Autodesk Inventor part; units mm, degrees
ref_plane "YZ Plane" through (0, 0, 0) normal (1, 0, 0) x (0, 1, 0)
ref_plane "XZ Plane" through (0, 0, 0) normal (0, 1, 0) x (-1, 0, 0)
ref_plane "XY Plane" through (0, 0, 0) normal (0, 0, 1) x (1, 0, 0)
sketch "Sketch1" plane through (0, 0, 0) normal (0, 0, 1) x (1, 0, 0)
  line L0 (0, 0) -> (80, 0)
  line L1 (80, 0) -> (80, 125.359)
  line L2 (60, 200) -> (80, 125.359)
  line L3 (60, 200) -> (137.2741, 200) construction
  line L4 (0, 0) -> (0, 125.359)
  line L5 (20, 200) -> (0, 125.359)
  line L6 (84, 125.8856) -> (84, -4)
  line L7 (84, -4) -> (-4, -4)
  line L8 (-4, -4) -> (-4, 125.8856)
  line L9 (-4, 125.8856) -> (16.9307, 204)
  line L10 (63.0693, 204) -> (84, 125.8856)
  line L11 (20, 204) -> (20, 200)
  line L12 (60, 200) -> (60, 204)
  line L13 (16.9307, 204) -> (20, 204)
  line L14 (60, 204) -> (63.0693, 204)
  point P0 (40, 0)
  dimension "d0" = 80
  dimension "d4" = 75
  dimension "d5" = 4
extrude "Extrusion1" add sketch "Sketch1" along normal blind 70
sketch "Sketch2" plane through (0, 0, 0) normal (0, 0, -1) x (-1, 0, 0)
  line L0 (-16.9307, 204) -> (4, 125.8856)
  line L1 (-84, 125.8856) -> (-63.0693, 204)
  line L2 (-16.9307, 204) -> (-63.0693, 204)
  line L3 (-80, 125.359) -> (-80, 0)
  line L4 (-60, 200) -> (-80, 125.359)
  line L5 (-60, 204) -> (-60, 200)
  line L6 (-63.0693, 204) -> (-60, 204)
  line L7 (-84, 125.8856) -> (-63.0693, 204)
  line L8 (-84, -4) -> (-84, 125.8856)
  line L9 (4, -4) -> (-84, -4)
  line L10 (4, 125.8856) -> (4, -4)
  line L11 (-16.9307, 204) -> (4, 125.8856)
  line L12 (-20, 204) -> (-16.9307, 204)
  line L13 (-20, 200) -> (-20, 204)
  line L14 (0, 125.359) -> (-20, 200)
  line L15 (0, 0) -> (0, 125.359)
  line L16 (-80, 0) -> (0, 0)
extrude "Extrusion2" add sketch "Sketch2" along normal blind 3
chamfer "Chamfer1" distance 5 angle 45 5 edges at (40, -4, -3) (84, 60.9428, -3) (-4, 60.9428, -3) (6.4653, 164.9428, -3) (73.5347, 164.9428, -3)
chamfer "Chamfer2" distance 3 angle 45 7 edges at (20, 202, 0) (10, 162.6795, 0) (60, 202, 0) (70, 162.6795, 0) (80, 62.6795, 0) (0, 62.6795, 0) (40, 0, 0)
chamfer "Chamfer3" distance 3 angle 45 4 edges at (84, -4, 36) (-4, -4, 36) (0, 0, 36.5) (80, 0, 36.5)
sketch "Sketch3" plane through (0, 0, 70) normal (0, 0, 1) x (1, 0, 0)
  line L0 (77, 0) -> (78.5, 1.5)
  line L1 (81, -4) -> (82.5, -2.5)
  line L2 (78.5, 1.5) -> (82.5, -2.5)
  line L3 (79, 1) -> (82.5, -2.5)
  circle A0 centre (80.75, -0.75) radius 1
  line L4 (-4, -1) -> (-2.5, -2.5)
  line L5 (-2.5, -2.5) -> (1.5, 1.5)
  line L6 (0, 3) -> (3, 0)
  line L7 (1, 1) -> (-2.5, -2.5)
  circle A1 centre (-0.75, -0.75) radius 1
  line L8 (3, 124.964) -> (0, 125.359)
  line L9 (16.9307, 204) -> (-4, 125.8856)
  line L10 (80, 125.359) -> (77, 124.964)
  line L11 (84, -1) -> (84, 125.8856)
  line L12 (1, 125.2273) -> (-4, 125.8856)
  circle A2 centre (82, 125.6223) radius 1
  circle A3 centre (-2, 125.6223) radius 1
  point P0 (0, 0)
  dimension "d19" = 2
  dimension "d20" = 2
  dimension "d22" = 2
  dimension "d23" = 2
extrude "Extrusion3" cut sketch "Sketch3" against normal blind 5
sketch "Sketch4" plane through (22.1071, 204, -3) normal (0, 1, 0) x (1, 0, 0)
  line L0 (35.7859, 0) -> (40.9622, -5)
  line L1 (38.374, -2.5) -> (36.3929, -4.5)
  line L2 (34.8929, -3) -> (37.8929, -6)
  circle A0 centre (37.3835, -3.5) radius 1
  line L3 (-21.1071, 0) -> (56.8929, 0)
  line L4 (17.8929, 0) -> (17.8929, -26)
  circle A1 centre (-1.5976, -3.5) radius 1
  point P0 (-22.1071, -3)
  dimension "d26" = 2
extrude "Extrusion4" cut sketch "Sketch4" against normal blind 15
sketch "Sketch5" plane through (0, 0, 0) normal (0, 0, 1) x (1, 0, 0)
  line L0 (77, 3) -> (3, 3)
  line L1 (40, 3) -> (40, 43)
  line L2 (40, 43) -> (40, 113)
  line L3 (40, 78) -> (20, 78)
  line L4 (20, 78) -> (20, 55.5)
  line L5 (20, 55.5) -> (60, 55.5)
  line L6 (60, 55.5) -> (60, 100.5)
  line L7 (60, 100.5) -> (20, 100.5)
  line L8 (20, 100.5) -> (20, 78)
  line L9 (40, 78) -> (70, 78)
  line L10 (70, 78) -> (70, 98)
  circle A0 centre (70, 98) radius 1
  line L11 (70, 78) -> (70, 58)
  circle A1 centre (70, 58) radius 1
  circle A2 centre (10, 98) radius 1
  circle A3 centre (10, 58) radius 1
  line L12 (40, 113) -> (40, 133)
  line L13 (40, 133) -> (63.1521, 133)
  line L14 (63.1521, 133) -> (63.1521, 155.7076)
  circle A4 centre (63.1521, 155.7076) radius 1.5
  circle A5 centre (63.1521, 133) radius 1.5
  circle A6 centre (16.8479, 155.7076) radius 1.5
  circle A7 centre (16.8479, 133) radius 1.5
  point P0 (0, 0)
  dimension "d29" = 40
  dimension "d30" = 70
  dimension "d31" = 20
  dimension "d32" = 22.5
  dimension "d33" = 40
  dimension "d34" = 45
  dimension "d35" = 30
  dimension "d36" = 20
  dimension "d37" = 2
  dimension "d38" = 20
  dimension "d39" = 2
  dimension "d40" = 20
  dimension "d41" = 23.1521
  dimension "d42" = 22.7076
  dimension "d43" = 3
  dimension "d44" = 3
extrude "Extrusion5" cut sketch "Sketch5" against normal blind 40
sketch "Sketch7" plane through (-1, -4, 2) normal (0, -1, 0) x (1, 0, 0)
  line L0 (78, 68) -> (4, 68)
  line L1 (41, 68) -> (41, 34)
  line L2 (54.7, 34) -> (27.3, 34)
  line L3 (54.7, 34) -> (54.7, 20.8)
  line L4 (54.7, 20.8) -> (27.3, 20.8)
  line L5 (27.3, 34) -> (27.3, 20.8)
  point P0 (1, -2)
  dimension "d47" = 27.4
  dimension "d48" = 34
  dimension "d49" = 13.2
extrude "Extrusion6" cut sketch "Sketch7" against normal blind 27.4
sketch "Sketch8" plane through (-4, 125.8856, 2) normal (-0.9659258, 0.258819, 0) x (0, 0, 1)
  line L0 (-2, 13.7678) -> (-2, 10.7678)
  line L1 (-2, 35.7017) -> (-2, 32.7017)
  line L2 (3.9828, 34.5121) -> (3.9828, 12.5782)
  line L3 (3.9828, 23.5451) -> (5.9828, 23.5451)
  line L4 (5.9828, 23.5451) -> (12.9828, 23.5451)
  line L5 (12.9828, 23.5451) -> (12.9828, 30.2951)
  line L6 (12.9828, 30.2951) -> (12.9828, 16.7951)
  line L7 (12.9828, 16.7951) -> (5.9828, 16.7951)
  line L8 (5.9828, 16.7951) -> (5.9828, 29.9848)
  line L9 (5.9828, 29.9848) -> (12.9828, 30.2951)
  point P0 (-2, -120.5609)
  point P1 (12.9828, 30.2951)
  dimension "d52" = 2
  dimension "d53" = 7
  dimension "d54" = 6.75
  dimension "d55" = 13.5
extrude "Extrusion7" cut sketch "Sketch8" against normal blind 9
chamfer "Chamfer4" distance 1 angle 45 4 edges at (5.7728, 154.6308, 14.9828) (2.2788, 141.5908, 14.9828) (2.2788, 141.5908, 7.9828) (5.6925, 154.331, 7.9828)
sketch "Sketch9" plane through (-4, 125.8856, 2) normal (-1, 0, 0) x (0, 0, 1)
  line L0 (1, -0.5266) -> (1, -122.8856)
  line L1 (1, -48.8247) -> (7.6436, -48.8247)
  line L2 (7.6436, -48.8247) -> (7.6436, -34.3247)
  line L3 (7.6436, -34.3247) -> (7.6436, -63.3247)
  circle A0 centre (7.6436, -34.3247) radius 2
  circle A1 centre (7.6436, -63.3247) radius 2
  point P0 (-2, -125.8856)
  dimension "d61" = 14.5
  dimension "d62" = 29
  dimension "d63" = 4
  dimension "d64" = 4
extrude "Extrusion8" cut sketch "Sketch9" against normal blind 999
sketch "Sketch17" plane through (0, 0, -3) normal (0, 0, -1) x (-1, 0, 0)
  line L0 (-60, 55.5) -> (-60, 100.5)
  line L1 (-60, 78) -> (-77, 78)
  line L2 (-77, 124.964) -> (-77, 3)
  line L3 (-77, 78) -> (-77, 43)
  line L4 (-77, 78) -> (-77, 113)
  line L5 (-60, 55.5) -> (-20, 55.5)
  line L6 (-40, 55.5) -> (-40, 37.7198)
  line L7 (-20, 55.5) -> (-20, 100.5)
  line L8 (-20, 78) -> (-3, 78)
  line L9 (-3, 78) -> (-3, 43)
  line L10 (-3, 78) -> (-3, 113)
  line L11 (-20, 55.5) -> (-60, 55.5)
  line L12 (-77, 43) -> (-3, 43)
  line L13 (-3, 3) -> (-3, 124.964)
  line L14 (-3, 113) -> (-77, 113)
  line L15 (-79, 1) -> (-79, 125.2273)
  circle A0 centre (-63.1521, 133) radius 1.5
  circle A1 centre (-70, 98) radius 1
  circle A2 centre (-10, 58) radius 1
  circle A3 centre (-16.8479, 133) radius 1.5
  circle A4 centre (-63.1521, 155.7076) radius 1.5
  circle A5 centre (-70, 58) radius 1
  circle A6 centre (-10, 98) radius 1
  circle A7 centre (-16.8479, 155.7076) radius 1.5
  line L16 (-20, 55.5) -> (-60, 55.5)
  line L17 (-60, 55.5) -> (-60, 100.5)
  line L18 (-60, 100.5) -> (-20, 100.5)
  line L19 (-20, 100.5) -> (-20, 55.5)
  line L20 (-79, 125.2273) -> (-57.8929, 204)
  line L21 (-79, 1) -> (-79, 125.2273)
  line L22 (-1, 1) -> (-79, 1)
  line L23 (-1, 125.2273) -> (-1, 1)
  line L24 (-22.1071, 204) -> (-1, 125.2273)
  line L25 (-22.1071, 204) -> (-57.8929, 204)
  point P0 (0, 0)
  dimension "d106" = 35
  dimension "d107" = 35
extrude "Extrusion16" add sketch "Sketch17" along normal blind 3 contours L5 L6 L12 L2 L1 L0 | L0 L18 L7 L5 | L1 L2 L14 L10 L8 L7 L18 L0 | L5 L7 L8 L9 L12 L6
sketch "Sketch18" plane through (0, 0, 70) normal (0, 0, 1) x (1, 0, 0)
  line L0 (-145.0841, -156.9657) -> (0, 339.906)
  line L1 (0, 339.906) -> (209.9789, 212.1699)
  line L2 (209.9789, 212.1699) -> (104.9894, -207.8436)
  line L3 (104.9894, -207.8436) -> (-145.0841, -156.9657)
  point P0 (0, 0)
extrude "Extrusion17" cut sketch "Sketch18" against normal blind 73
sketch "Sketch19" plane through (0, 0, -3) normal (0, 0, 1) x (1, 0, 0)
  line L0 (3, 113) -> (77, 113)
  line L1 (77, 43) -> (3, 43)
  line L2 (40, 43) -> (40, 113)
  line L3 (40, 78) -> (25, 78)
  line L4 (25, 78) -> (25, 63)
  line L5 (25, 63) -> (40, 63)
  line L6 (40, 63) -> (55, 63)
  line L7 (55, 63) -> (55, 93)
  line L8 (55, 93) -> (25, 93)
  line L9 (25, 93) -> (25, 78)
  line L10 (22, 78) -> (22, 60)
  line L11 (22, 60) -> (40, 60)
  line L12 (40, 60) -> (58, 60)
  line L13 (58, 60) -> (58, 96)
  line L14 (58, 96) -> (22, 96)
  line L15 (22, 96) -> (22, 78)
  point P0 (0, 0)
  dimension "d112" = 15
  dimension "d113" = 15
  dimension "d114" = 15
  dimension "d115" = 15
  dimension "d116" = 30
  dimension "d117" = 3
extrude "Extrusion18" add sketch "Sketch19" along normal blind 73 contours L11 L10 L15 L14 L2 L8 L9 L4 L5 | L2 L6 L7 L8 L14 L13 L12
sketch "Sketch20" plane through (0, 0, -3) normal (0, 0, 1) x (1, 0, 0)
  line L0 (25, 93) -> (25, 63)
  line L1 (25, 63) -> (55, 63)
  line L2 (55, 63) -> (55, 93)
  line L3 (55, 93) -> (25, 93)
  point P0 (0, 0)
extrude "Extrusion19" cut sketch "Sketch20" against normal blind 73
chamfer "Chamfer7" distance 3 angle 45 8 edges at (58, 60, 33.5) (25, 93, 32) (58, 96, 33.5) (55, 63, 32) (22, 96, 33.5) (55, 93, 32) (25, 63, 32) (22, 60, 33.5)
chamfer "Chamfer8" distance 3 angle 45 4 edges at (3, 78, -3) (40, 43, -3) (77, 78, -3) (40, 113, -3)
sketch "Sketch21" plane through (25, 96, -3) normal (0, 1, 0) x (1, 0, 0)
  line L0 (0, -73) -> (0, 0)
  line L1 (30, -73) -> (0, -73)
  line L2 (30, 0) -> (30, -73)
  line L3 (0, 0) -> (30, 0)
  line L4 (0, -73) -> (0, 3)
  line L5 (0, -35) -> (30, -35)
  line L6 (30, -73) -> (30, 0)
  circle A0 centre (15, -35) radius 9.425
  point P0 (-25, -3)
  dimension "d128" = 18.85
extrude "Extrusion20" cut sketch "Sketch21" against normal blind 3 contours A0 L5 | L5 A0
sketch "Sketch22" plane through (0, 0, 70) normal (0, 0, 1) x (1, 0, 0)
  line L0 (25, 60) -> (22, 63)
  line L1 (25, 60) -> (55, 60)
  line L2 (58, 63) -> (55, 60)
  line L3 (58, 63) -> (58, 93)
  line L4 (55, 96) -> (58, 93)
  line L5 (55, 96) -> (25, 96)
  line L6 (22, 93) -> (25, 96)
  line L7 (22, 93) -> (22, 63)
  line L8 (28, 93) -> (52, 93)
  line L9 (55, 90) -> (52, 93)
  line L10 (55, 90) -> (55, 66)
  line L11 (52, 63) -> (55, 66)
  line L12 (52, 63) -> (28, 63)
  line L13 (25, 66) -> (28, 63)
  line L14 (25, 66) -> (25, 90)
  line L15 (28, 93) -> (25, 90)
  line L16 (25, 90) -> (28, 93)
  line L17 (26.5, 91.5) -> (23.5, 94.5)
  line L18 (22, 93) -> (25, 96)
  line L19 (25, 60) -> (22, 63)
  line L20 (23.5, 61.5) -> (26.5, 64.5)
  line L21 (28, 63) -> (25, 66)
  line L22 (56.5, 61.5) -> (53.5, 64.5)
  line L23 (53.5, 91.5) -> (56.5, 94.5)
  line L24 (58, 93) -> (55, 96)
  circle A0 centre (25, 63) radius 1
  circle A1 centre (55, 63) radius 1
  circle A2 centre (55, 93) radius 1
  circle A3 centre (25, 93) radius 1
  point P0 (0, 0)
  dimension "d131" = 2
  dimension "d132" = 2
  dimension "d133" = 2
  dimension "d134" = 2
extrude "Extrusion21" cut sketch "Sketch22" against normal blind 20 contours A0 L20 | L20 A0 | A1 L22 | L22 A1 | A3 L17 | L17 A3 | A2 L23 | L23 A2
equation "\"d45\" = d33"
equation "\"d50\" = d47"
properties part number "the handle"
Model file for the job. Use its own axes, mm. A direction names the side the tool comes from. Coordinates: 2 decimals unless noted, no trailing zeros. Loops run counter-clockwise (first coordinate to the right, second up) from the corner with the lowest first, then second, coordinate; pieces in that order, holes last. Notation, with made-up numbers: (63.25, 75) - (117.25, 75) arc R15 cw to (117.25, 86) - close; hole circle Ø7 at (73, 26). An arc over 180 degrees is marked (long way). Answer as a JSON object with one key per item and string values. Group by question number.
(1) Cut at C-C (z = 55). Give the cut face in (x, y), then the cut area to 3 significant figures.
(2) Flat gauge pins, fed straight in: pin 1 (1.2 mm diameter, centred on x = 55, y = 63, fed in from +Z); pin 2 (15 mm diameter, centred on x = 42.5, z = 30.5, fed in from -Y); pin 3 (7 mm diameter, centred on y = 74, z = 14.5, fed in from +X); pin 4 (1.6 mm diameter, centred on x = 10, y = 98, fed in from -Z). Where does each tip first touch, or does it go through?
(3) Cut at B-B (x = 40). State how many separate pieces and enclosed holes the cut face has, then the cut area to 3 significant figures.
(4) Tool access for faces 4 (the face through (55, 78, 33)), 5 (the face through (56, 95, 34)), 6 (the face through (5, 78, -4)), 7 (the face through (25, 93, 50)), 8 (the face through (39, 111, -4)): list every direction of +Z, -Z, +X, -X, +Y, -Y with a clear straight run to the whole face (end or side of a thin tool).
(5) Two-plate mould, pull along X, no slides. Class faces 1 (the face through (54, 91, 31)), 2 (the face through (22, 78, 33)), 3 (the face through (41, 94, -6)): released by +X, released by -X, zero draft, split by the parting line, or undercut.
(6) Probe line 1 along Y through (x, z) = (32, 57); line 2 along X through (y, z) = (73, 15.5); line 3 along Y through (x, z) = (70, -5). List the from-to ranges inside material, lowest first.
Geometry says:
{
 "1": {"outline": "(22, 63) - (25, 60) - (55, 60) - (58, 63) - (58, 93) - (55, 96) - (25, 96) - (22, 93) - close; hole circle Ø2 at (25, 63); hole circle Ø2 at (25, 93); hole (25, 66) - (28, 63) - (52, 63) - (55, 66) - (55, 90) - (52, 93) - (28, 93) - (25, 90) - close; hole circle Ø2 at (55, 63); hole circle Ø2 at (55, 93)", "area": "383 mm^2"},
 "2": {"pin 1": "stops at z = 50", "pin 2": "stops at y = 60", "pin 3": "stops at x = 58", "pin 4": "passes through"},
 "3": {"separate pieces": "3", "enclosed holes": "0", "area": "492 mm^2"},
 "4": {"face 4": "+Z, -Z", "face 5": "+Z, +X, +Y", "face 6": "+Z, -X, +Y, -Y", "face 7": "+Z", "face 8": "+Z, +X, -X, +Y"},
 "5": {"face 1": "undercut", "face 2": "released by -X", "face 3": "zero draft"},
 "6": {"line 1": "y = 60 to 63, 93 to 96", "line 2": "x = 22 to 25, 55 to 58", "line 3": "y = 44 to 57, 59 to 97, 99 to 112"}
}
